Job drawing, mm, ordinate dimensions from the low corner. One solid piece. A direction names the side the tool comes from. Give positions to 0.01 mm unless a question says otherwise; leave off trailing zeros. Loops run counter-clockwise (first coordinate to the right, second up) from the corner with the lowest first, then second, coordinate; pieces in that order, holes last. Notation, with made-up numbers: (37.25, 41) - (42.25, 41) arc R5 cw to (42.25, 45) - close; hole circle Ø11 at (54, 46.25). An arc over 180 degrees is marked (long way). Use a Markdown table: item, result.
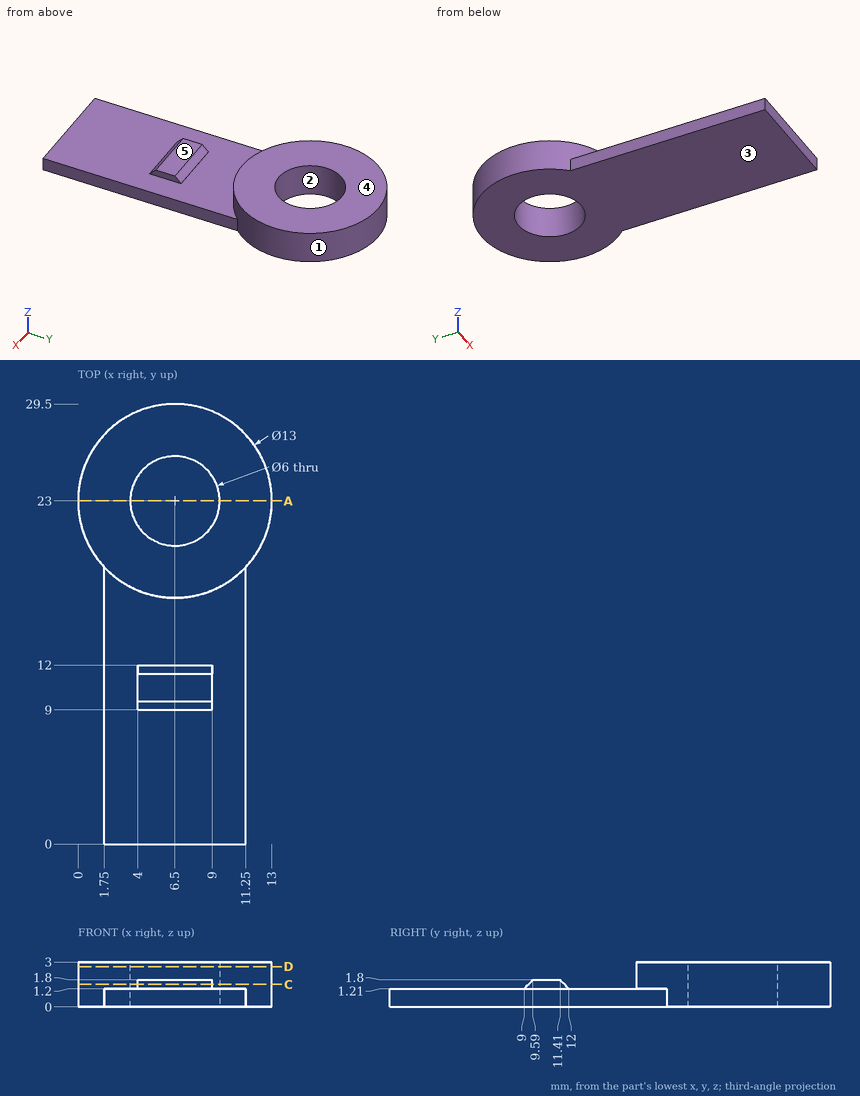
(1) Slice it at C-C, the plane z = 1.5. Write the cut outline in (x, y).
Computed:
| item | result |
|---|---|
| outline | circle Ø13 at (6.5, 23); (4, 9.29) - (9, 9.29) - (9, 11.71) - (4, 11.71) - close; hole circle Ø6 at (6.5, 23) |
(2) 3-axis set-ups, long thin cutter, end or side, ignore diameter. For the marked faces 4 and 5: which of +Z, -Z, +X, -X, +Y, -Y reach the whole face in a straight line?
Computed:
| item | result |
|---|---|
| face 4 | +Z, +X, -X, +Y, -Y |
| face 5 | +Z, +X, -X, -Y |
(3) Pin check, flat tips, straight feed: P1, Ø6, axis at x = 11, y = 19.5, coming from the -Z side; P2, Ø1.5, axis at x = 6, y = 14.5, coming from the +Z side; P3, Ø1.3, axis at y = 13.5, z = 0.5, coming from the -X side; P4, Ø5, axis at x = 5.5, y = 7, coming from the +Z side. Stop position of each tip, or through.
Computed:
| item | result |
|---|---|
| P1 | z = 0 |
| P2 | z = 1.2 |
| P3 | x = 1.75 |
| P4 | z = 1.71 |
(4) Drill centre lines: probe 1 along Y at (x, z) = (6.5, 1.15); probe 2 along Y at (x, z) = (6.5, 1.4); probe 3 along Y at (x, z) = (6.5, 1.6). Where is each one in solid material? Low to high. Write a range as [from, to].
Computed:
| item | result |
|---|---|
| probe 1 | [0, 20], [26, 29.5] |
| probe 2 | [9.19, 11.81], [16.5, 20], [26, 29.5] |
| probe 3 | [9.39, 11.61], [16.5, 20], [26, 29.5] |
(5) Mould opens along X. For the marked faces 1, 2 and 3 say: pulls with the +X half, pulls with the -X half, needs draft (parallel to the pull), parting line crosses it, or undercut.
Computed:
| item | result |
|---|---|
| face 1 | parting line crosses it |
| face 2 | undercut |
| face 3 | needs draft |
(6) Slice it at D-D, the plane z = 2.7. Write the cut outline in (x, y), plus the area to 3 significant figures.
Computed:
| item | result |
|---|---|
| outline | circle Ø13 at (6.5, 23); hole circle Ø6 at (6.5, 23) |
| area | 104 mm² |
(7) Slice it at A-A, the plane y = 23. Write the cut outline in (x, z).
Computed:
| item | result |
|---|---|
| outline | (0, 0) - (3.5, 0) - (3.5, 3) - (0, 3) - close; (9.5, 0) - (13, 0) - (13, 3) - (9.5, 3) - close |
